Geometry: see drawing. Coordinates: mm, zero at the bounding-box minimum. Give positions to 0.01 mm unless a question says otherwise; leave off trailing zeros. Order: outer loops, then holes, each group sorted by start corner. A loop starts at its lowest first (then second) coordinate and runs counter-clockwise, first axis right, second up. Notation, with made-up numbers: M 5,-32 L 30,-32 A15 ccw 30,-24 Z; hole C 35,-34.5 d3. An arc over 180 degrees is marked long. Return JSON: item names as keys, results as strings.
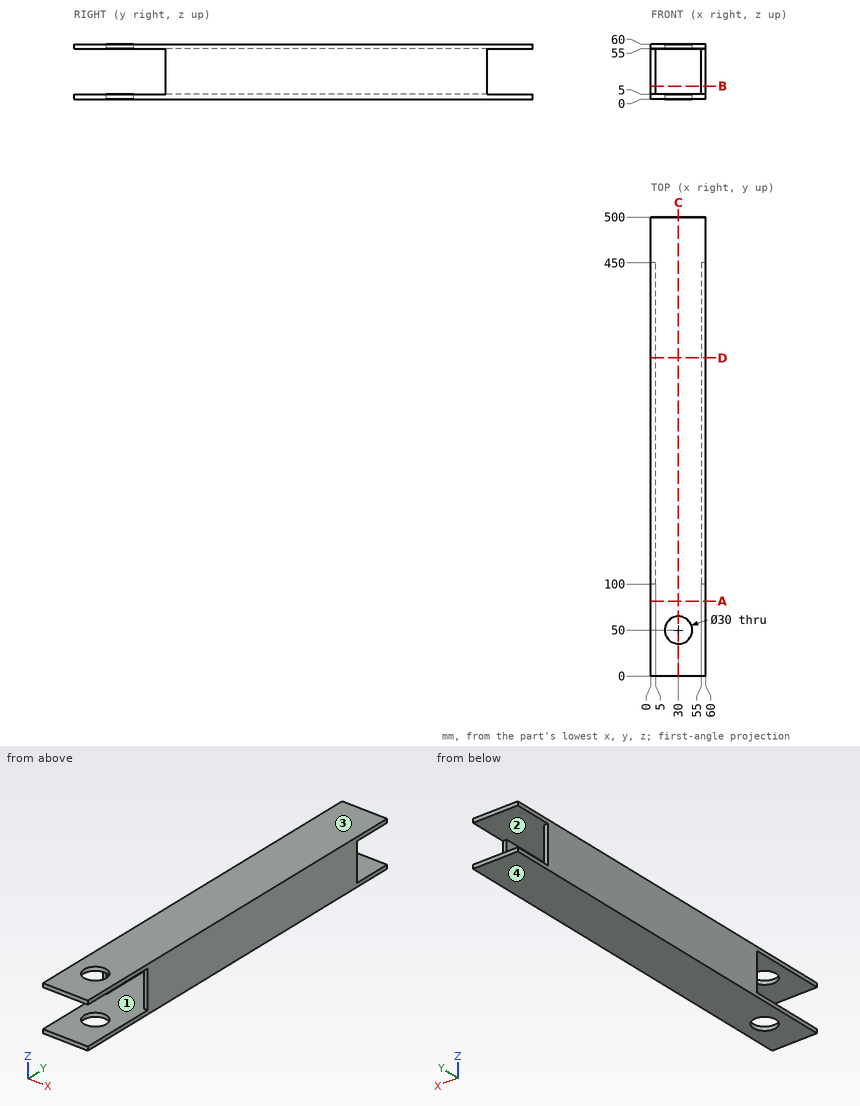
1. Section query C-C (x = 30). Return loops of the section in (y, z).
Evaluation:
{"outline": "M 0,0 L 35,0 L 35,5 L 0,5 Z; M 0,55 L 35,55 L 35,60 L 0,60 Z; M 65,0 L 500,0 L 500,5 L 65,5 Z; M 65,55 L 500,55 L 500,60 L 65,60 Z"}
2. Draft query along Z for the marked faces 1, 2, 3 and 4. Return one class per face: pulls with the +Z half, pulls with the -Z half, needs draft (parallel to the pull), parting line crosses it, or undercut.
Evaluation:
{"face 1": "undercut", "face 2": "undercut", "face 3": "pulls with the +Z half", "face 4": "pulls with the -Z half"}
3. Ray query, probe 1 along Z at (x, y) = (53.5, 449); probe 2 along Y at (x, z) = (30, 2). Return the intervals inside material, ascending.
Evaluation:
{"probe 1": "z = 0 to 5, 55 to 60", "probe 2": "y = 0 to 35, 65 to 500"}
4. First-contact query: pin 1 (24 mm diameter, centred on x = 30, y = 50, fed in from +Z); pin 2 (1.5 mm diameter, centred on x = 3.5, z = 22, fed in from -Y); pin 3 (1.5 mm diameter, centred on x = 3, z = 40.5, fed in from +Y). Flat tips, straight axial feed; report the tip coordinate or a pass-through.
Evaluation:
{"pin 1": "passes through", "pin 2": "stops at y = 100", "pin 3": "stops at y = 450"}
5. Section query A-A (y = 81.5). Return loops of the section in (x, z).
Evaluation:
{"outline": "M 0,0 L 60,0 L 60,5 L 0,5 Z; M 0,55 L 60,55 L 60,60 L 0,60 Z"}
6. Section query B-B (z = 14). Return loops of the section in (x, y), then the cut area to 3 significant figures.
Evaluation:
{"outline": "M 0,100 L 5,100 L 5,450 L 0,450 Z; M 55,100 L 60,100 L 60,450 L 55,450 Z", "area": "3,500 mm^2"}
7. Section query D-D (y = 346.5). Return loops of the section in (x, z), then the cut area to 3 significant figures.
Evaluation:
{"outline": "M 0,0 L 60,0 L 60,60 L 0,60 Z; hole M 5,5 L 55,5 L 55,55 L 5,55 Z", "area": "1,100 mm^2"}
